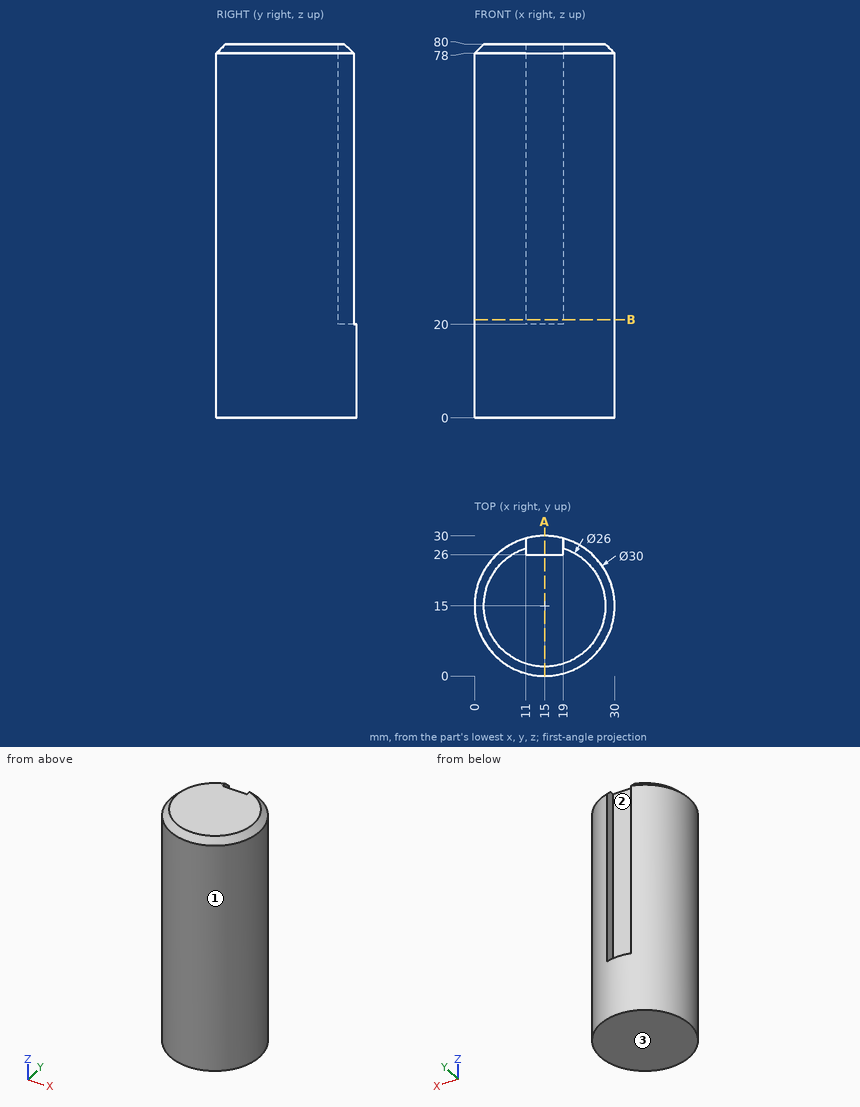
Answer from the drawing. Dimensions are ordinates in mm from the lowest x, y and z of the part. Give positions to 0.01 mm unless a question says otherwise; leave off trailing zeros. Write each loop counter-clockwise with the first axis right and the second up, starting at its lowest first coordinate (ties: lowest second). Pieces come first, ordered by that corner, then holes. Notation, with made-up numbers: (-10.75, -24.5) - (37.25, -24.5) arc R15 cw to (37.25, -18.5) - close; hole circle Ø6 at (85.5, -20.75). An arc over 180 degrees is marked (long way). One line per item, written item: value. Start each with the question number.
1. For a pull along X with two mould halves and no side action, classify the marked faces 1, 2 and 3 as +X half, -X half, draft (parallel to the pull), parting line (faces both ways), or undercut.
2. Consider probe 1 along Y at (x, z) = (7.5, 38.5); probe 2 along Y at (x, z) = (15, 51); probe 3 along X at (y, z) = (26.75, 47.5). Determine where each line is inside the solid, lowest interval first.
3. Given pin 1 (6 mm diameter, centred on x = 10.5, z = 17.5, fed in from -Y); pin 2 (3 mm diameter, centred on y = 27.5, z = 54, fed in from -X); pin 3 (1.7 mm diameter, centred on y = 28, z = 57, fed in from +X), each flat-ended and moving along its own axis, determine where each tip first touches the part or whether it passes through.
4. Find section B-B (z = 21). Write down the section's boundary in (x, y).
5. Find section A-A (x = 15). Write down the section's boundary in (y, z).
Geometry results:
1. face 1: parting line
1. face 2: undercut
1. face 3: draft
2. probe 1: 2.01 to 27.99
2. probe 2: 0 to 26
2. probe 3: 5.68 to 11, 19 to 24.32
3. pin 1: y = 0.08
3. pin 2: x = 4.8
3. pin 3: x = 23.8
4. outline: (11, 26) - (11, 29.46) arc R15 ccw (long way) to (19, 29.46) - (19, 26) - close
5. outline: (0, 0) - (30, 0) - (30, 20) - (26, 20) - (26, 80) - (2, 80) - (0, 78) - close
